```python
from build123d import *

# Parameters (mm, degrees)
F0_R     = 38.1
F1_DEPTH = 25.4
F2_R     = 6.35
F3_DEPTH = 12.7
F4_R     = 4.7625
F5_DEPTH = 12.7


with BuildPart() as f1:
    # F0 (on Front) → F1 (new body)
    with BuildSketch(Plane.XZ):
        Circle(F0_R)
    extrude(amount=F1_DEPTH)

    # F2 (on face) → F3 (cut)
    with BuildSketch(Plane.XZ.offset(25.4)):
        Circle(F2_R)
    extrude(amount=-F3_DEPTH, mode=Mode.SUBTRACT)

    # F4 (on face) → F5 (cut)
    with BuildSketch(Plane(origin=(0, 0, 0), x_dir=(-1, 0, 0), z_dir=(0, 1, 0))):
        with Locations((0, 28.575)):
            Circle(F4_R)
    extrude(amount=-F5_DEPTH, mode=Mode.SUBTRACT)


solid = f1.part
```
The listing builds one solid part. Answer for the finished solid, in the listing's coordinates (mm). A direction names the side the tool comes from. Give positions to 0.01 mm unless a question says otherwise; leave off trailing zeros. Order: outer loops, then holes, each group sorted by start corner. A loop starts at its lowest first (then second) coordinate and runs counter-clockwise, first axis right, second up.
Item 1: The part is cut by section D-D, the plane y = -6. Give the vertices of the cut face in (x, z) (1 decimal), and give its area (3 significant figures).
From the geometry:
outline: circle Ø76.2 at (0, 0); hole circle Ø9.5 at (0, 28.6)
area: 4,490 mm2
Item 2: For a pull along X with two mould halves and no side action, classify faces 4 (the face through (8, -25.4, 1)), 5 (the face through (-1.38, -19.14, -6.2)), 6 (the face through (-30.235, -12.522, -23.183)) as pulls with the +X half, pulls with the -X half, needs draft (parallel to the pull), parting line crosses it, or undercut.
From the geometry:
face 4: needs draft
face 5: undercut
face 6: parting line crosses it
Item 3: The part is cut by section A-A, the plane z = 0. Give the vertices of the cut face in (x, y), and give its area (3 significant figures).
From the geometry:
outline: (-38.1, -25.4) - (-6.35, -25.4) - (-6.35, -12.7) - (6.35, -12.7) - (6.35, -25.4) - (38.1, -25.4) - (38.1, 0) - (-38.1, 0) - close
area: 1,770 mm2
Item 4: The part is cut by section C-C, the plane y = -16.25. Give the vertices of the cut face in (x, z).
From the geometry:
outline: circle Ø76.2 at (0, 0); hole circle Ø12.7 at (0, 0)
Item 5: Given pin 1 Ø8 at (y, z) = (-17.5, 29.5) entering from +X; pin 2 Ø1.5 at (y, z) = (-22, -7) entering from -X; pin 3 Ø3 at (y, z) = (-21.5, -16.5) entering from +X, each flat-ended and moving along its own axis, determine where each tip first touches the part or whether it passes through.
From the geometry:
pin 1: stops at x = 28.31
pin 2: stops at x = -37.58
pin 3: stops at x = 35.02
Item 6: Which of the six approach directions +Z, -Z, +X, -X, +Y, -Y give full straight-line access (tool end or side, diameter ignored) to faces 1 (the face through (-1, 0, 1)), 2 (the face through (0, -12.7, 29)), 3 (the face through (0, -12.7, 0))?
From the geometry:
face 1: +Z, -Z, +X, -X, +Y
face 2: +Y
face 3: -Y
Item 7: The part is cut by section B-B, the plane x = 0. Give the vertices of the cut face in (y, z).
From the geometry:
outline: (-25.4, -38.1) - (0, -38.1) - (0, 23.81) - (-12.7, 23.81) - (-12.7, 33.34) - (0, 33.34) - (0, 38.1) - (-25.4, 38.1) - (-25.4, 6.35) - (-12.7, 6.35) - (-12.7, -6.35) - (-25.4, -6.35) - close
Item 8: Find the intervals of material crossed by probe 1 along Z at (x, y) = (0, -9); probe 2 along Z at (x, y) = (0, -21.5); probe 3 along X at (y, z) = (-20, 0.5), in increasing order.
From the geometry:
probe 1: z = -38.1 to 23.81, 33.34 to 38.1
probe 2: z = -38.1 to -6.35, 6.35 to 38.1
probe 3: x = -38.1 to -6.33, 6.33 to 38.1
